Design review of the part shown in the three views and the two pictorial views. Dimensions are in mm from the part's minimum x, y and z. A direction names the side the tool comes from. Round coordinates to 2 decimals unless told otherwise and drop trailing zeros. Order: outer loops, then holes, each group sorted by start corner. A loop starts at its lowest first (then second) coordinate and runs counter-clockwise, first axis right, second up.
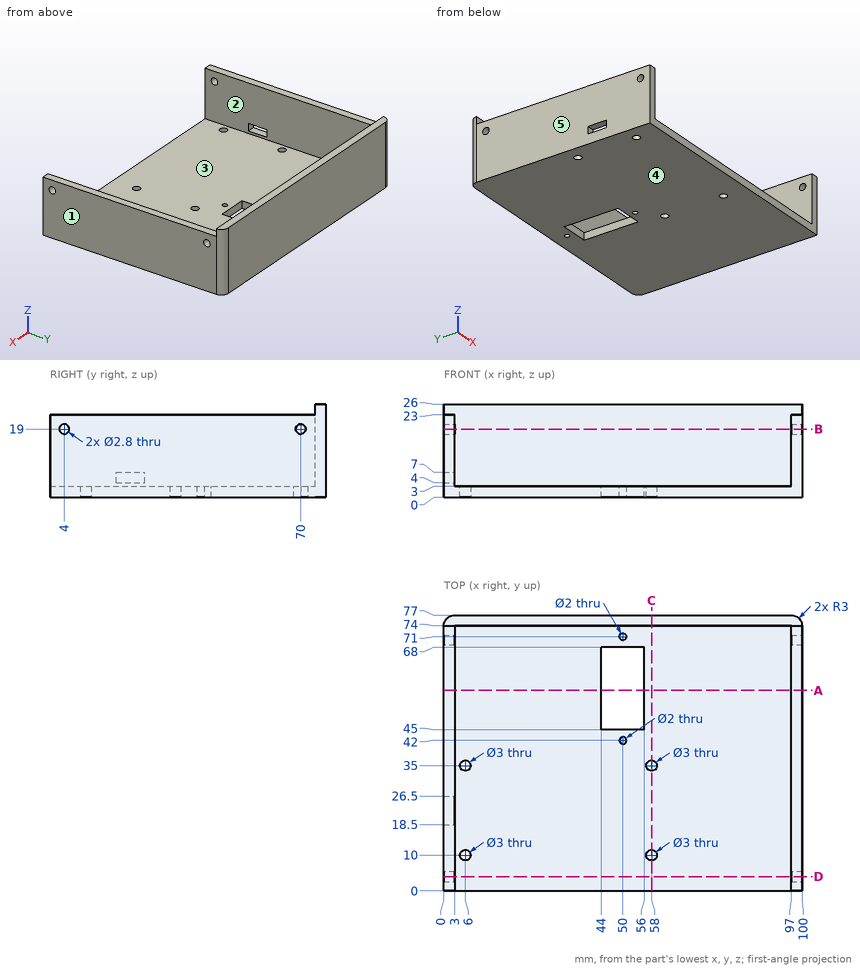
1) Clearance check with flat-ended pins moving along their axes: P1, Ø1.5, axis at x = 69.5, z = 16.5, coming from the -Y side; P2, Ø2.5, axis at x = 1, z = 5.5, coming from the +Y side; P3, Ø4, axis at x = 58, y = 35, coming from the +Z side. State where each tip first meets the part, or that it passes through.
Results:
P1: stops at y = 74
P2: stops at y = 76.9
P3: stops at z = 3
2) Take a section at A-A on y = 56. Give the boundary of the cut face in (x, z).
Results:
outline: (0, 0) - (44, 0) - (44, 3) - (3, 3) - (3, 23) - (0, 23) - close; (56, 0) - (100, 0) - (100, 23) - (97, 23) - (97, 3) - (56, 3) - close
3) Take a section at B-B on z = 19. Give the boundary of the cut face in (x, y).
Results:
outline: (0, 0) - (3, 0) - (3, 2.6) - (0, 2.6) - close; (0, 5.4) - (3, 5.4) - (3, 68.6) - (0, 68.6) - close; (0, 71.4) - (3, 71.4) - (3, 74) - (97, 74) - (97, 71.4) - (100, 71.4) - (100, 74) arc R3 ccw to (97, 77) - (3, 77) arc R3 ccw to (0, 74) - close; (97, 0) - (100, 0) - (100, 2.6) - (97, 2.6) - close; (97, 5.4) - (100, 5.4) - (100, 68.6) - (97, 68.6) - close
4) Take a section at C-C on x = 58. Give the boundary of the cut face in (y, z), plus the area to 3 significant figures.
Results:
outline: (0, 0) - (8.5, 0) - (8.5, 3) - (0, 3) - close; (11.5, 0) - (33.5, 0) - (33.5, 3) - (11.5, 3) - close; (36.5, 0) - (77, 0) - (77, 26) - (74, 26) - (74, 3) - (36.5, 3) - close
area: 282 mm2
5) Take a section at D-D on y = 4. Give the boundary of the cut face in (x, z), plus the area to 3 significant figures.
Results:
outline: (0, 0) - (100, 0) - (100, 17.6) - (97, 17.6) - (97, 3) - (3, 3) - (3, 17.6) - (0, 17.6) - close; (0, 20.4) - (3, 20.4) - (3, 23) - (0, 23) - close; (97, 20.4) - (100, 20.4) - (100, 23) - (97, 23) - close
area: 403 mm2
6) To check wall thickness, follow line 1 along X through (y, z) = (56, 9.5); line 2 along Z through (x, y) = (98, 70); line 3 along Z through (x, y) = (34, 69). State the ranges of each line that lie inside material, in increasing order.
Results:
line 1: x = 0 to 3, 97 to 100
line 2: z = 0 to 17.6, 20.4 to 23
line 3: z = 0 to 3
7) The part is to be moulded in two halves that separate along X. For the marked faces 3, 4 and 5, say which applies: released by +X, released by -X, zero draft, split by the parting line, or undercut.
Results:
face 3: undercut
face 4: zero draft
face 5: released by -X
8) For the marked faces 1 and 2, list the 3-axis set-ups (+Z, -Z, +X, -X, +Y, -Y) from which the entire face can be reached by the end or side of a thin tool; tool diameter is ignored.
Results:
face 1: +Z, -Z, +X, +Y, -Y
face 2: +Z, -Y
